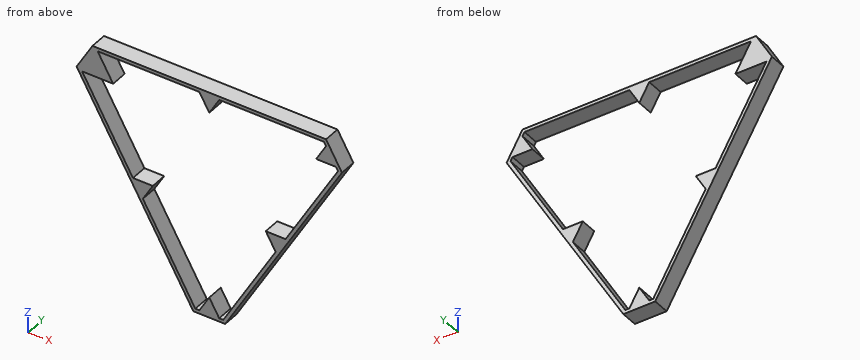
from build123d import *

# Parameters (mm, degrees)
BOSS_EXTRUDE1_DEPTH = 12.38


with BuildPart() as part:
    # Sketch1 → Boss-Extrude1 (new body)
    with BuildSketch(Plane(origin=(0, 0, 0), x_dir=(1, 0, 0), z_dir=(0, 1, 0))):
        Polygon((-11.732050803, 167.865334802), (11.732050803, 167.865334802), (97.741669748, 18.89230485), (86.00961895, -1.428203229), (-86.009618944, -1.428203229), (-97.741669751, 18.892304845), align=None)
        Polygon((41.607695163, 85.798692796), (56.226497316, 85.798692796), (94.854918412, 18.892304841), (93.36528139, 16.312177834), (78.746479233, 16.312177834), (86.055880312, 3.651923793), (84.566243293, 1.071796793), (7.309401088, 1.071796793), (2e-09, 13.732050847), (-7.309401083, 1.071796796), (-82.256842179, 1.071796796), (-70.813466519, 20.892304849), (-93.70021784, 20.892304849), (-56.226497283, 85.798692801), (-41.60769513, 85.798692801), (-48.917096207, 98.458946839), (-10.288675112, 165.365334792), (-7.309401077, 165.365334792), (0, 152.705080754), (7.309401077, 165.365334792), (10.288675142, 165.365334792), (48.91709624, 98.458946834), align=None, mode=Mode.SUBTRACT)
    extrude(amount=BOSS_EXTRUDE1_DEPTH)


solid = part.part
Work out the finished part from the listing and answer in its coordinate system (mm). Coordinates: 2 decimals unless noted, no trailing zeros. Loops run counter-clockwise (first coordinate to the right, second up) from the corner with the lowest first, then second, coordinate; pieces in that order, holes last. Notation, with made-up numbers: (38, -37.75) -> (68, -37.75) arc R16 cw to (68, -29.75) -> close; hole circle Ø11 at (88, 19). An arc over 180 degrees is marked (long way). Answer as CSV lines item,"result".
1) The part is cut by section C-C (z = -66). Give the vertices of the cut face in (x, y).
A:
outline,"(-70.54, 0) -> (-67.66, 0) -> (-67.66, 12.38) -> (-70.54, 12.38) -> close; (67.66, 0) -> (70.54, 0) -> (70.54, 12.38) -> (67.66, 12.38) -> close"
2) The part is cut by section B-B (y = 5.75). Give the vertices of the cut face in (x, z), and give its area (3 significant figures).
A:
outline,"(-97.74, -18.89) -> (-11.73, -167.87) -> (11.73, -167.87) -> (97.74, -18.89) -> (86.01, 1.43) -> (-86.01, 1.43) -> close; hole (-93.7, -20.89) -> (-56.23, -85.8) -> (-41.61, -85.8) -> (-48.92, -98.46) -> (-10.29, -165.37) -> (-7.31, -165.37) -> (0, -152.71) -> (7.31, -165.37) -> (10.29, -165.37) -> (48.92, -98.46) -> (41.61, -85.8) -> (56.23, -85.8) -> (94.85, -18.89) -> (93.37, -16.31) -> (78.75, -16.31) -> (86.06, -3.65) -> (84.57, -1.07) -> (7.31, -1.07) -> (0, -13.73) -> (-7.31, -1.07) -> (-82.26, -1.07) -> (-70.81, -20.89) -> close"
area,"2,180 mm²"
3) The part is cut by section A-A (x = 52). Give the vertices of the cut face in (y, z), and give its area (3 significant figures).
A:
outline,"(0, -98.12) -> (12.38, -98.12) -> (12.38, -85.8) -> (0, -85.8) -> close; (0, -1.07) -> (12.38, -1.07) -> (12.38, 1.43) -> (0, 1.43) -> close"
area,"183 mm²"
4) Flat-ended cylindrical pins translate along their axes: pin 1 (1.5 mm diameter, centred on x = -17, y = 5.5, fed in from -Z); pin 2 (3 mm diameter, centred on x = 47, y = 1.5, fed in from -Z); pin 3 (1 mm diameter, centred on x = 14, y = 3, fed in from -Z). Find the tip coordinate at first contact, or state that the pin passes through.
A:
pin 1,"stops at z = -160.04"
pin 2,"stops at z = -109.38"
pin 3,"stops at z = -164.8"
5) Straight lines are drawn through the part: probe 1 along Z at (x, y) = (-10, 5.75); probe 2 along X at (y, z) = (10.5, -153); probe 3 along X at (y, z) = (8.25, -11.5). For each, find the intervals that lie inside material, in ascending order.
A:
probe 1,"z = -167.87 to -165.37, -1.07 to 1.43"
probe 2,"x = -20.31 to -17.43, -0.17 to 0.17, 17.43 to 20.31"
probe 3,"x = -93.47 to -76.24, -1.29 to 1.29, 81.52 to 93.47"
